Answer from the drawing. Dimensions are ordinates in mm from the lowest x, y and z of the part. A direction names the side the tool comes from. Round coordinates to 2 decimals unless told otherwise and drop trailing zeros. Order: outer loops, then holes, each group sorted by start corner. A loop starts at its lowest first (then second) coordinate and runs counter-clockwise, first axis right, second up.
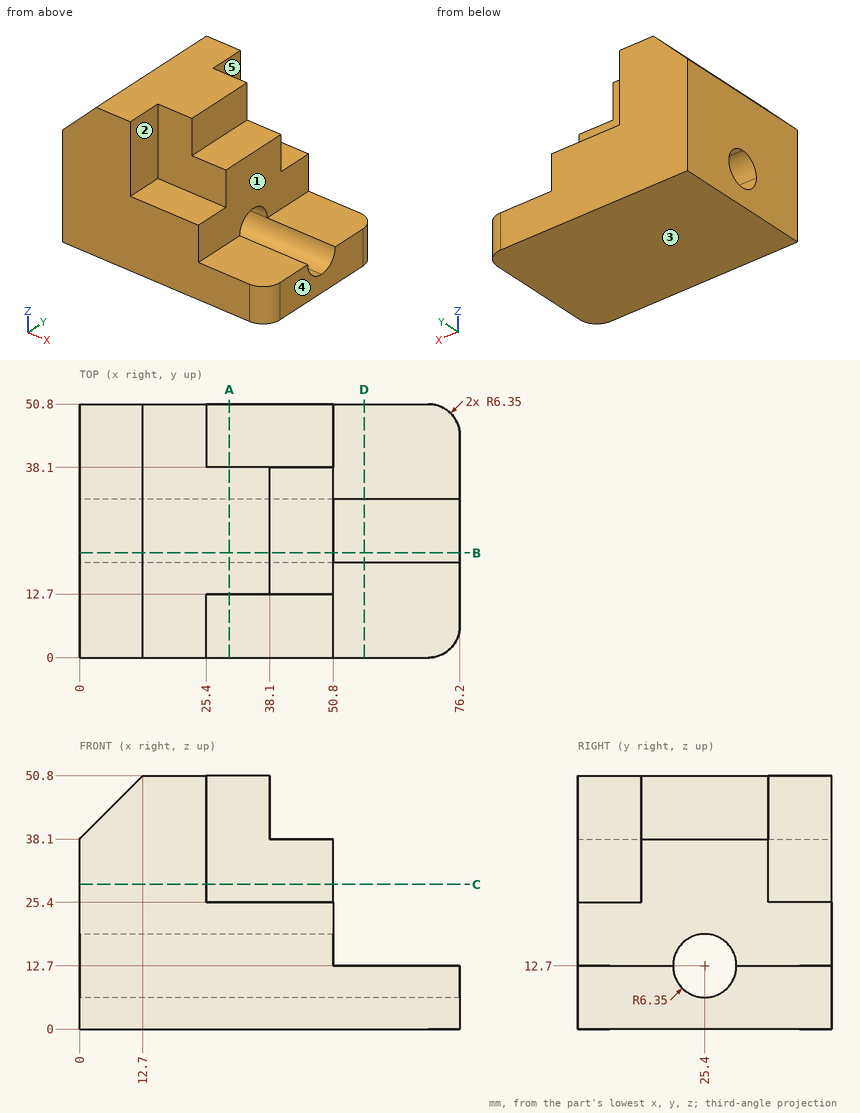
Q1. A cutting plane is placed at B-B, the plane y = 21. Give the vertices of the cut face in (x, z).
Outcome:
outline: (0, 0) - (76.2, 0) - (76.2, 8.12) - (0, 8.12) - close; (0, 17.28) - (50.8, 17.28) - (50.8, 38.1) - (38.1, 38.1) - (38.1, 50.8) - (12.7, 50.8) - (0, 38.1) - close
Q2. A cutting plane is placed at D-D, the plane x = 57. Give the vertices of the cut face in (y, z).
Outcome:
outline: (0, 0) - (50.8, 0) - (50.8, 12.7) - (31.75, 12.7) arc R6.35 cw to (19.05, 12.7) - (0, 12.7) - close
Q3. Flat-ended cylindrical pins translate along their axes: pin 1 (10 mm diameter, centred on y = 20.5, z = 42.5, fed in from +X); pin 2 (15 mm diameter, centred on x = 65.5, y = 6, fed in from +Z); pin 3 (4 mm diameter, centred on x = 36.5, y = 7, fed in from +Z). Find the tip coordinate at first contact, or state that the pin passes through.
Outcome:
pin 1: stops at x = 50.8
pin 2: stops at z = 12.7
pin 3: stops at z = 25.4
Q4. A cutting plane is placed at C-C, the plane z = 29. Give the vertices of the cut face in (x, y).
Outcome:
outline: (0, 0) - (25.4, 0) - (25.4, 12.7) - (50.8, 12.7) - (50.8, 38.1) - (25.4, 38.1) - (25.4, 50.8) - (0, 50.8) - close
Q5. For the marked faces 1, 2, 3, 4 and 5, determine the directions among +Z, -Z, +X, -X, +Y, -Y from which every point of the face is accessible in a straight line to the end or side of a thin tool.
Outcome:
face 1: +Z, +X, +Y, -Y
face 2: +Z, +X, -Y
face 3: -Z, +X, -X, +Y, -Y
face 4: +Z, -Z, +X, +Y, -Y
face 5: +Z, +X, +Y
Q6. Straight lines are drawn through the part: probe 1 along Y at (x, z) = (28.5, 13); probe 2 along X at (y, z) = (33, 18.5); probe 3 along Z at (x, y) = (72, 7). For each, find the intervals that lie inside material, in ascending order.
Outcome:
probe 1: y = 0 to 19.06, 31.74 to 50.8
probe 2: x = 0 to 50.8
probe 3: z = 0 to 12.7
Q7. A cutting plane is placed at A-A, the plane x = 30. Give the vertices of the cut face in (y, z).
Outcome:
outline: (0, 0) - (50.8, 0) - (50.8, 25.4) - (38.1, 25.4) - (38.1, 50.8) - (12.7, 50.8) - (12.7, 25.4) - (0, 25.4) - close; hole circle Ø12.7 at (25.4, 12.7)
